Here's how the part is built. I have some questions about the finished solid (model axes, mm). Face numbers are marked on the shaded views. A direction names the side the tool comes from. Coordinates: 2 decimals unless noted, no trailing zeros. Order: outer loops, then holes, each group sorted by start corner. A loop starts at its lowest first (then second) coordinate and runs counter-clockwise, first axis right, second up.
```python
from build123d import *

# Parameters (mm, degrees)
PAD_DEPTH       = 36
SKETCH001_W     = 41.77589
SKETCH001_H     = 47.890068
POCKET_DEPTH    = 10.5
SKETCH002_R     = 2.75
POCKET001_DEPTH = 36.001
FILLET_R        = 4
FILLET001_R     = 0.5
SKETCH003_R     = 2.85
HOLE_DEPTH      = 16.001
FILLET002_R     = 4
CHAMFER_SIZE    = 2
POCKET002_DEPTH = 3
FILLET003_R     = 2


with BuildPart() as part:
    # Sketch → Pad (new body)
    with BuildSketch(Plane.XZ):
        with BuildLine():
            Line((-30.008135, 0), (9.991865, 0))
            Line((9.991865, 10), (9.991865, 0))
            Line((10, 10), (9.991865, 10))
            Line((10, 30), (10, 10))
            ThreePointArc((10, 30), (0, 40), (-10, 30))
            Line((-10, 10), (-10, 30))
            Line((-30.008135, 10), (-10, 10))
            Line((-30.008135, 0), (-30.008135, 10))
        make_face()
    extrude(amount=PAD_DEPTH)

    # Sketch001 (on DatumPlane) → Pocket (cut, symmetric)
    with BuildSketch(Plane(origin=(0, -18, 0), x_dir=(1, 0, 0), z_dir=(0, 1, 0))):
        with Locations((0.131337, -38.945034)):
            Rectangle(SKETCH001_W, SKETCH001_H)
    extrude(amount=POCKET_DEPTH, both=True, mode=Mode.SUBTRACT)

    # Sketch002 (on Face4 of Pocket) → Pocket001 (cut, through all)
    with BuildSketch(Plane(origin=(0, 0, 0), x_dir=(1, 0, 0), z_dir=(0, 1, 0))):
        with Locations((0, -30)):
            Circle(SKETCH002_R)
    extrude(amount=-POCKET001_DEPTH, mode=Mode.SUBTRACT)

    # Fillet
    fillet_edges = [part.edges().sort_by_distance(p)[0] for p in [
        (10, -18, 15),
        (-10, -18, 15),
    ]]
    fillet(fillet_edges, radius=FILLET_R)

    # Fillet001
    fillet001_edges = [part.edges().sort_by_distance(p)[0] for p in [
        (-10, -18, 10),
    ]]
    fillet(fillet001_edges, radius=FILLET001_R)

    # Sketch003 (on DatumPlane) → Hole (cut, through all)
    with BuildSketch(Plane(origin=(0, 0, 16), x_dir=(1, 0, 0), z_dir=(0, 0, -1))):
        with Locations((4.991865, 18)):
            Circle(SKETCH003_R)
        with Locations((-25.008135, 18)):
            Circle(SKETCH003_R)
    extrude(amount=HOLE_DEPTH, mode=Mode.SUBTRACT)

    # Fillet002
    fillet002_edges = [part.edges().sort_by_distance(p)[0] for p in [
        (-30.008135, 0, 5),
        (-30.008135, -36, 5),
    ]]
    fillet(fillet002_edges, radius=FILLET002_R)

    # Chamfer
    chamfer_edges = [part.edges().sort_by_distance(p)[0] for p in [
        (-2.75, 0, 30),
    ]]
    chamfer(chamfer_edges, length=CHAMFER_SIZE)

    # Sketch004 (on Face14 of Chamfer) → Pocket002 (cut)
    with BuildSketch(Plane.XZ.offset(36)):
        Polygon((-0.093793, 34.5), (-3.944011, 32.168773), (-3.850218, 27.668773), (0.093793, 25.5), (3.944011, 27.831227), (3.850218, 32.331227), align=None)
    extrude(amount=-POCKET002_DEPTH, mode=Mode.SUBTRACT)

    # Fillet003
    fillet003_edges = [part.edges().sort_by_distance(p)[0] for p in [
        (10, 0, 20),
        (10, -36, 20),
    ]]
    fillet(fillet003_edges, radius=FILLET003_R)


solid = part.part
```
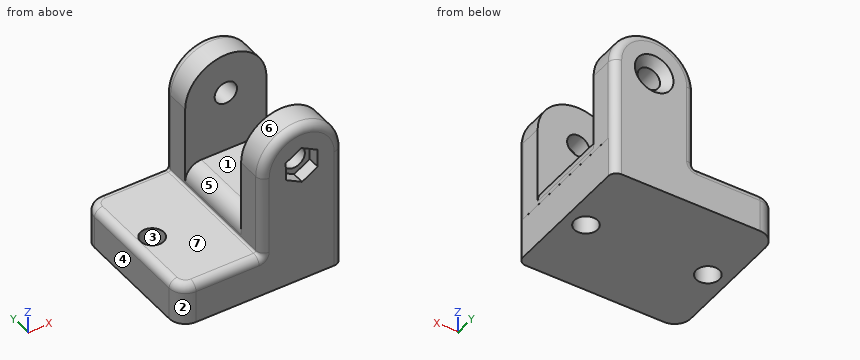
Q1. If we section it at B-B on x = -13.5: Write out the boundary of the cut face in (y, z), then the cut area to 3 significant figures.
Q2. If we section it at D-D on y = -18: Give the number of separate pieces and of enclosed holes in the cut face, then the cut area to 3 significant figures.
Q3. For the marked faces 5, 6 and 7, which set-ups out of +Z, -Z, +X, -X, +Y, -Y let a thin tool reach every point of the face, with its end or its side?
Q4. I need wall thicknesses on L1, parallel to Y at x = 5.5, z = 31.5; L2, parallel to X at y = -32, z = 30; L3, parallel to Z at x = 0, y = -4. Which ranges of each line are inside material? Lowest first, please.
Q5. Will these pins go through, and if not, where does the flat tip stop? pin 1 (22 mm diameter, centred on x = 1.5, z = 32.5, fed in from +Y); pin 2 (3.5 mm diameter, centred on x = 4.99, y = -18, fed in from +Z); pin 3 (7 mm diameter, centred on x = 0, z = 30, fed in from +Y); pin 4 (1 mm diameter, centred on y = -30, z = 27, fed in from -X).
Q6. We'd pull the mould along Y, two halves only. Please class the marked faces 1, 2, 3 and 4: pulls with the +Y half, pulls with the -Y half, needs draft (parallel to the pull), parting line crosses it, or undercut.
Reply:
1. outline: (-36, 0) - (0, 0) - (0, 8) arc R2 ccw to (-2, 10) - (-34, 10) arc R2 ccw to (-36, 8) - close
1. area: 358 mm2
2. separate pieces: 3
2. enclosed holes: 0
2. area: 350 mm2
3. face 5: +Z, -X
3. face 6: +Z, +Y, -Y
3. face 7: +Z, -X, +Y, -Y
4. L1: y = -36 to -28.5, -7.5 to 0
4. L2: x = -10 to -2.75, 2.75 to 10
4. L3: z = 0 to 27.25, 32.75 to 40
5. pin 1: stops at y = 0
5. pin 2: passes through
5. pin 3: stops at y = -1.25
5. pin 4: stops at x = -10
6. face 1: undercut
6. face 2: pulls with the -Y half
6. face 3: undercut
6. face 4: needs draft
